```python
from build123d import *

# Parameters (mm, degrees)
F1_DEPTH = 10
F3_DEPTH = 5
F5_DEPTH = 25.4
F6_R     = 6.34999
F8_DEPTH = 5
F9_DEPTH = 25.4


# Not quite as in the source:
# - a fillet or chamfer is up to 0.001 mm smaller than in the source, because OpenCascade refuses the exact size


with BuildPart() as f1:
    # F0 (on Top) → F1 (new body)
    with BuildSketch(Plane.XY):
        with BuildLine():
            ThreePointArc((46.5285696909, 5.9739645023), (0, 40.5641849146), (-46.5285696909, 5.9739645023))
            ThreePointArc((-46.5285696909, 5.9739645023), (-49.6833366753, -30.6579453037), (-41.1537964933, -66.4224013325))
            ThreePointArc((-41.1537964933, -66.4224013325), (-34.8569562758, -98.8847496511), (-41.1537964933, -131.3470979697))
            ThreePointArc((-41.1537964933, -131.3470979697), (-44.1025989066, -166.693183735), (-30.5410850268, -199.467053752))
            ThreePointArc((-30.5410850268, -199.467053752), (0, -213.4927201844), (30.5410850268, -199.467053752))
            ThreePointArc((30.5410850268, -199.467053752), (44.1025989066, -166.693183735), (41.1537964933, -131.3470979697))
            ThreePointArc((41.1537964933, -131.3470979697), (34.8569562758, -98.8847496511), (41.1537964933, -66.4224013325))
            ThreePointArc((41.1537964933, -66.4224013325), (49.6833366753, -30.6579453037), (46.5285696909, 5.9739645023))
        make_face()
    extrude(amount=F1_DEPTH)

    # F2 (on face) → F3 (cut)
    with BuildSketch(Plane.XY.offset(10)):
        with BuildLine():
            Line((31.75, -5.715), (0, -5.715))
            Line((0, -5.715), (0, -18.415))
            Line((0, -18.415), (-19.05, -18.415))
            ThreePointArc((-19.05, -18.415), (-22.7697438789, -27.3952561211), (-31.75, -31.115))
            Line((-31.75, -31.115), (31.75, -31.115))
            ThreePointArc((31.75, -31.115), (19.05, -18.415), (31.75, -5.715))
        make_face()
        with BuildLine():
            Line((0, -18.415), (0, -5.715))
            Line((0, -5.715), (-31.75, -5.715))
            ThreePointArc((-31.75, -5.715), (-22.7697438789, -9.4347438789), (-19.05, -18.415))
            Line((-19.05, -18.415), (0, -18.415))
        make_face()
        with BuildLine():
            ThreePointArc((-19.05, -18.415), (-22.7697438789, -9.4347438789), (-31.75, -5.715))
            ThreePointArc((-31.75, -5.715), (-44.45, -18.415), (-31.75, -31.115))
            ThreePointArc((-31.75, -31.115), (-22.7697438789, -27.3952561211), (-19.05, -18.415))
        make_face()
        with BuildLine():
            ThreePointArc((44.45, -18.415), (40.7302561211, -9.4347438789), (31.75, -5.715))
            ThreePointArc((31.75, -5.715), (19.05, -18.415), (31.75, -31.115))
            ThreePointArc((31.75, -31.115), (40.7302561211, -27.3952561211), (44.45, -18.415))
        make_face()
    extrude(amount=-F3_DEPTH, mode=Mode.SUBTRACT)

    # F4 (on face) → F5 (cut)
    with BuildSketch(Plane.XY.offset(5)):
        Polygon((-31.75, -12.065), (-31.75, -18.415), (-31.75, -24.765), (31.75, -24.765), (31.75, -12.065), align=None)
    extrude(amount=-F5_DEPTH, mode=Mode.SUBTRACT)

    # F6 (radius 6.35 in the source; OpenCascade refuses exactly that, so slightly less here)
    f6_edges = [f1.edges().sort_by_distance(p)[0] for p in [
        (-31.75, -12.065, 2.5),
        (-31.75, -24.765, 2.5),
        (31.75, -12.065, 2.5),
        (31.75, -24.765, 2.5),
    ]]
    fillet(f6_edges, radius=F6_R)

    # F7 (on face) → F8 (cut)
    with BuildSketch(Plane.XY.offset(10)):
        with BuildLine():
            Line((25.4, -148.9900371552), (-25.4, -148.9900371552))
            ThreePointArc((-25.4, -148.9900371552), (-38.1, -161.6900371552), (-25.4, -174.3900371552))
            Line((-25.4, -174.3900371552), (25.4, -174.3900371552))
            ThreePointArc((25.4, -174.3900371552), (38.1, -161.6900371552), (25.4, -148.9900371552))
        make_face()
        with BuildLine():
            ThreePointArc((-15.24, -167.4590520005), (-21.59, -161.1090520005), (-15.24, -154.7590520005))
            Line((-15.24, -154.7590520005), (15.24, -154.7590520005))
            ThreePointArc((15.24, -154.7590520005), (21.59, -161.1090520005), (15.24, -167.4590520005))
            Line((15.24, -167.4590520005), (-15.24, -167.4590520005))
        make_face(mode=Mode.SUBTRACT)
    extrude(amount=-F8_DEPTH, mode=Mode.SUBTRACT)

    # F9 (cut): a face of the model
    f9_faces = [f1.faces().sort_by_distance(p)[0] for p in [
        (0, -161.1090520005, 10),
    ]]
    extrude(f9_faces, amount=-F9_DEPTH, mode=Mode.SUBTRACT)


solid = f1.part
```
CAD build for the part. Positions are in the model's coordinates, mm. A direction names the side the tool comes from. Coordinates: 2 decimals unless noted, no trailing zeros. Order: outer loops, then holes, each group sorted by start corner. A loop starts at its lowest first (then second) coordinate and runs counter-clockwise, first axis right, second up. Notation, with made-up numbers: (42.25, 43) -> (70.25, 43) arc R24 ccw to (70.25, 73) -> close; hole circle Ø2 at (27, 30). An arc over 180 degrees is marked (long way). Use one line per item in the form item = value. Start each with the question number.
1) Drop flat-ended pins along their axis: pin 1 (1.5 mm diameter, centred on x = 11, z = 7, fed in from -Y); pin 2 (5 mm diameter, centred on y = -169.5, z = 8, fed in from +X); pin 3 (1.5 mm diameter, centred on x = -5, z = 2, fed in from -Y). Give the stop position or say it passes through.
2) Band-saw the part on B-B on y = -172. Give the cut face in (x, z).
3) Band-saw the part on D-D on y = -42. Give the cut face in (x, z).
4) Drill centre lines: L1, parallel to Y at x = -9, z = 1.75 (3 decimals); L2, parallel to Y at x = 6.5, z = 9.25 (3 decimals); L3, parallel to Z at x = -31.5, y = -168.5. Where is each one in solid material? Low to high. Write a range as [from, to].
5) Band-saw the part on C-C on y = 2. Give the cut face in (x, z).
6) Band-saw the part on A-A on z = 7.5. State how many separate pieces and enclosed holes the cut face has, then the cut area to 3 significant figures.
7) Pull direction X, two halves, no side cores. Call faces 4 (the cylindrical face through (-34.86, -98.42, 4.93)), 5 (the flat face through (-1, -170, 5)), 6 (the cylindrical face through (-0.49, -213.49, 4.93)): +X half, -X half, draft (parallel to the pull), parting line (faces both ways), or undercut.
8) Tool access for faces 1 (the flat face through (-1, -85, 10)), 2 (the flat face through (0, -31.115, 8)), 3 (the cylindrical face through (29.84, -22.954, 2.465)): list every direction of +Z, -Z, +X, -X, +Y, -Y with a clear straight run to the whole face (end or side of a thin tool).
Entries:
q1.pin_1 = -212.17
q1.pin_2 = 44.05
q1.pin_3 = -213.27
q2.outline = (-43.08, 0) -> (43.08, 0) -> (43.08, 10) -> (32.82, 10) -> (32.82, 5) -> (-32.82, 5) -> (-32.82, 10) -> (-43.08, 10) -> close
q3.outline = (-48.27, 0) -> (48.27, 0) -> (48.27, 10) -> (-48.27, 10) -> close
q4.L1 = [-212.474, -167.459], [-154.759, -24.765], [-12.065, 39.723]
q4.L2 = [-212.965, -174.39], [-148.99, -31.115], [-5.715, 40.127]
q4.L3 = [0, 5]
q5.outline = (-47.45, 0) -> (47.45, 0) -> (47.45, 10) -> (-47.45, 10) -> close
q6.separate_pieces = 1
q6.enclosed_holes = 2
q6.area = 16,400 mm2
q7.face_4 = -X half
q7.face_5 = undercut
q7.face_6 = parting line
q8.face_1 = +Z, +X, -X, +Y, -Y
q8.face_2 = +Z
q8.face_3 = +Z, -Z
